```python
from build123d import *

# Parameters (mm, degrees)
SKETCH1_W           = 84
SKETCH1_H           = 21
SKETCH1_W_2         = 80
SKETCH1_H_2         = 17
SKETCH1_W_3         = 6
SKETCH1_H_3         = 12
SKETCH1_H_4         = 4
SKETCH1_W_4         = 46
BOSS_EXTRUDE1_DEPTH = 2
SKETCH1_4_W         = 84
SKETCH1_4_H         = 21
SKETCH1_4_W_2       = 80
SKETCH1_4_H_2       = 17
SKETCH1_4_W_3       = 6
SKETCH1_4_H_3       = 12
SKETCH1_4_H_4       = 4
BOSS_EXTRUDE2_DEPTH = 11
SKETCH2_W           = 6
SKETCH2_H           = 3
SKETCH2_H_2         = 11
CUT_EXTRUDE1_DEPTH  = 9
SKETCH3_W           = 18
SKETCH3_H           = 9
CUT_EXTRUDE2_DEPTH  = 2
SKETCH4_W           = 4
SKETCH4_H           = 4
BOSS_EXTRUDE3_DEPTH = 9
SKETCH5_R           = 0.5
SKETCH5_R_2         = 1.5
CUT_EXTRUDE3_DEPTH  = 1
CUT_EXTRUDE4_DEPTH  = 24


with BuildPart() as part:
    # Sketch1 → Boss-Extrude1 (new body)
    # profile 1 of 7: a face of its own
    with BuildSketch(Plane(origin=(0, 0, 0), x_dir=(1, 0, 0), z_dir=(0, 1, 0))):
        Polygon((38, 10.5), (42, 10.5), (42, 12.5), (62, 12.5), (62, 13.5), (62, 14.5), (41, 14.5), align=None)
    # profile 2 of 7: a face of its own
    with BuildSketch(Plane(origin=(0, 0, 0), x_dir=(1, 0, 0), z_dir=(0, 1, 0))):
        Rectangle(SKETCH1_W, SKETCH1_H)
        Rectangle(SKETCH1_W_2, SKETCH1_H_2, mode=Mode.SUBTRACT)
    # profile 3 of 7: a face of its own
    with BuildSketch(Plane(origin=(0, 0, 0), x_dir=(1, 0, 0), z_dir=(0, 1, 0))):
        with Locations((-37, -2.5)):
            Rectangle(SKETCH1_W_3, SKETCH1_H_3)
    # profile 4 of 7: a face of its own
    with BuildSketch(Plane(origin=(0, 0, 0), x_dir=(1, 0, 0), z_dir=(0, 1, 0))):
        Polygon((-34, -8.5), (-14, -8.5), (-14, 3.5), (-8, 3.5), (-8, 4.5), (-14, 4.5), (-14, 8.5), (-34, 8.5), (-34, 4.5), (-40, 4.5), (-40, 4.448678332), (-40, 3.5), (-34, 3.5), align=None)
    # profile 5 of 7: a face of its own
    with BuildSketch(Plane(origin=(0, 0, 0), x_dir=(1, 0, 0), z_dir=(0, 1, 0))):
        with Locations((-37, 6.5)):
            Rectangle(SKETCH1_W_3, SKETCH1_H_4)
    # profile 6 of 7: a face of its own
    with BuildSketch(Plane(origin=(0, 0, 0), x_dir=(1, 0, 0), z_dir=(0, 1, 0))):
        Polygon((-14, -8.5), (-6, -8.5), (-6, 8.5), (-14, 8.5), (-14, 4.5), (-8, 4.5), (-8, 3.5), (-14, 3.5), align=None)
    # profile 7 of 7: a face of its own
    with BuildSketch(Plane(origin=(0, 0, 0), x_dir=(1, 0, 0), z_dir=(0, 1, 0))):
        with Locations((17, 0)):
            Rectangle(SKETCH1_W_4, SKETCH1_H_2)
    extrude(amount=BOSS_EXTRUDE1_DEPTH)

    # Sketch1_4 → Boss-Extrude2 (add)
    # profile 1 of 5: a face of its own
    with BuildSketch(Plane(origin=(0, 0, 0), x_dir=(1, 0, 0), z_dir=(0, 1, 0))):
        Polygon((38, 10.5), (42, 10.5), (42, 12.5), (62, 12.5), (62, 13.5), (62, 14.5), (41, 14.5), align=None)
    # profile 2 of 5: a face of its own
    with BuildSketch(Plane(origin=(0, 0, 0), x_dir=(1, 0, 0), z_dir=(0, 1, 0))):
        Rectangle(SKETCH1_4_W, SKETCH1_4_H)
        Rectangle(SKETCH1_4_W_2, SKETCH1_4_H_2, mode=Mode.SUBTRACT)
    # profile 3 of 5: a face of its own
    with BuildSketch(Plane(origin=(0, 0, 0), x_dir=(1, 0, 0), z_dir=(0, 1, 0))):
        Polygon((-14, -8.5), (-6, -8.5), (-6, 8.5), (-14, 8.5), (-14, 4.5), (-8, 4.5), (-8, 3.5), (-14, 3.5), align=None)
    # profile 4 of 5: a face of its own
    with BuildSketch(Plane(origin=(0, 0, 0), x_dir=(1, 0, 0), z_dir=(0, 1, 0))):
        with Locations((-37, -2.5)):
            Rectangle(SKETCH1_4_W_3, SKETCH1_4_H_3)
    # profile 5 of 5: a face of its own
    with BuildSketch(Plane(origin=(0, 0, 0), x_dir=(1, 0, 0), z_dir=(0, 1, 0))):
        with Locations((-37, 6.5)):
            Rectangle(SKETCH1_4_W_3, SKETCH1_4_H_4)
    extrude(amount=BOSS_EXTRUDE2_DEPTH)

    # Sketch2 → Cut-Extrude1 (cut)
    with BuildSketch(Plane(origin=(0, 11, 0), x_dir=(1, 0, 0), z_dir=(0, 1, 0))):
        with Locations((-37, 7)):
            Rectangle(SKETCH2_W, SKETCH2_H)
        with Locations((-37, -3)):
            Rectangle(SKETCH2_W, SKETCH2_H_2)
    extrude(amount=-CUT_EXTRUDE1_DEPTH, mode=Mode.SUBTRACT)

    # Sketch3 → Cut-Extrude2 (cut)
    with BuildSketch(Plane(origin=(0, 0, -10.5), x_dir=(-1, 0, 0), z_dir=(0, 0, -1))):
        with Locations((31, 6.5)):
            Rectangle(SKETCH3_W, SKETCH3_H)
    extrude(amount=-CUT_EXTRUDE2_DEPTH, mode=Mode.SUBTRACT)

    # Sketch4 → Boss-Extrude3 (add)
    with BuildSketch(Plane(origin=(0, 2, 0), x_dir=(1, 0, 0), z_dir=(0, 1, 0))):
        with Locations((0, 6.5)):
            Rectangle(SKETCH4_W, SKETCH4_H)
        with Locations((0, -6.5)):
            Rectangle(SKETCH4_W, SKETCH4_H)
        with Locations((34, 6.5)):
            Rectangle(SKETCH4_W, SKETCH4_H)
        with Locations((34, -6.5)):
            Rectangle(SKETCH4_W, SKETCH4_H)
    extrude(amount=BOSS_EXTRUDE3_DEPTH)

    # Sketch5 → Cut-Extrude3 (cut)
    # profile 1 of 2: a face of its own
    with BuildSketch(Plane(origin=(0, 0, -14.5), x_dir=(-1, 0, 0), z_dir=(0, 0, -1))):
        with BuildLine():
            Line((-62, 8), (-62, 5.5))
            Line((-62, 5.5), (-62, 3))
            Line((-62, 3), (-53.5, 4))
            ThreePointArc((-53.5, 4), (-55, 5.5), (-53.5, 7))
            Line((-53.5, 7), (-62, 8))
        make_face()
        with Locations((-58.5, 5.5)):
            Circle(SKETCH5_R, mode=Mode.SUBTRACT)
        with Locations((-56, 5.5)):
            Circle(SKETCH5_R, mode=Mode.SUBTRACT)
    # profile 2 of 2: a face of its own
    with BuildSketch(Plane(origin=(0, 0, -14.5), x_dir=(-1, 0, 0), z_dir=(0, 0, -1))):
        with Locations((-53.5, 5.5)):
            Circle(SKETCH5_R_2)
        with Locations((-53.5, 5.5)):
            Circle(SKETCH5_R, mode=Mode.SUBTRACT)
    extrude(amount=-CUT_EXTRUDE3_DEPTH, mode=Mode.SUBTRACT)

    # Sketch6 → Cut-Extrude4 (cut)
    with BuildSketch(Plane(origin=(62, 0, 0), x_dir=(0, 0, -1), z_dir=(1, 0, 0))):
        Polygon((10.5, 11), (14.5, 11), (14.5, 9), align=None)
        Polygon((10.5, 0), (14.5, 2), (14.5, 0), align=None)
    extrude(amount=-CUT_EXTRUDE4_DEPTH, mode=Mode.SUBTRACT)


solid = part.part
```
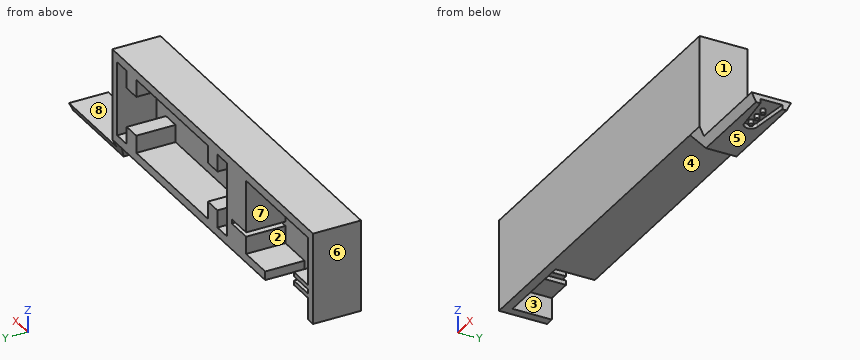
Work out the finished part from the listing and answer in its coordinate system (mm). Face numbers are marked on the shaded views. A direction names the side the tool comes from. Round coordinates to 2 decimals unless told otherwise and drop trailing zeros. Loops run counter-clockwise (first coordinate to the right, second up) from the corner with the lowest first, then second, coordinate; pieces in that order, holes last.
(1) The part is cut by section D-D, the plane x = -23.5. Give the vertices of the cut face in (y, z), and give its area (3 significant figures).
Computed values:
outline: (0, -10.5) - (2, -10.5) - (2, 8.5) - (11, 8.5) - (11, 10.5) - (0, 10.5) - close
area: 60.0 mm2
(2) The part is cut by section C-C, the plane x = 33. Give the vertices of the cut face in (y, z).
Computed values:
outline: (0, -10.5) - (11, -10.5) - (11, -4.5) - (2, -4.5) - (2, 4.5) - (11, 4.5) - (11, 10.5) - (0, 10.5) - close
(3) For the marked faces 1, 2, 3 and 4, determine the directions among +Z, -Z, +X, -X, +Y, -Y from which every point of the face is accessible in a straight line to the end or side of a thin tool.
Computed values:
face 1: +Z, +X, +Y, -Y
face 2: +Y
face 3: -Z, +Y
face 4: -Z, -X, +Y, -Y
(4) The part is cut by section A-A, the plane x = -13. Give the vertices of the cut face in (y, z), and give its area (3 significant figures).
Computed values:
outline: (0, -10.5) - (11, -10.5) - (11, -4.5) - (2, -4.5) - (2, -3.5) - (11, -3.5) - (11, 10.5) - (0, 10.5) - close
area: 222 mm2
(5) Each of these flat-tipped pins is pushed along its axis until it touches: P1, Ø2.5, axis at y = 5, z = -8.5, coming from the +X side; P2, Ø2, axis at x = 30, z = -4, coming from the +Y side; P3, Ø3, axis at x = -0.5, y = 5.5, coming from the -Z side. Where does it stop, or does it pass through?
Computed values:
P1: stops at x = 42
P2: stops at y = 2
P3: stops at z = -10.5
(6) The part is cut by section B-B, the plane z = 3. Give the vertices of the cut face in (x, y), and give its area (3 significant figures).
Computed values:
outline: (-42, 0) - (42, 0) - (42, 11) - (40, 11) - (40, 2) - (-6, 2) - (-6, 11) - (-14, 11) - (-14, 2) - (-40, 2) - (-40, 11) - (-42, 11) - close
area: 276 mm2
(7) The mould has two halves that part along Z. Classify the marked faces 5, 6, 7 and 8: pulls with the +Z half, pulls with the -Z half, needs draft (parallel to the pull), parting line crosses it, or undercut.
Computed values:
face 5: pulls with the -Z half
face 6: needs draft
face 7: undercut
face 8: pulls with the +Z half
(8) Find the intervals of material crossed by L1, parallel to X at y = 4, z = 3; L2, parallel to X at y = 9.25, z = -7.25; L3, parallel to X at y = 8.5, z = -3, in increasing order.
Computed values:
L1: x = -42 to -40, -14 to -6, 40 to 42
L2: x = -42 to -40, -14 to -6, -2 to 2, 32 to 36, 40 to 42
L3: x = -42 to -34, -14 to -6, 40 to 42
